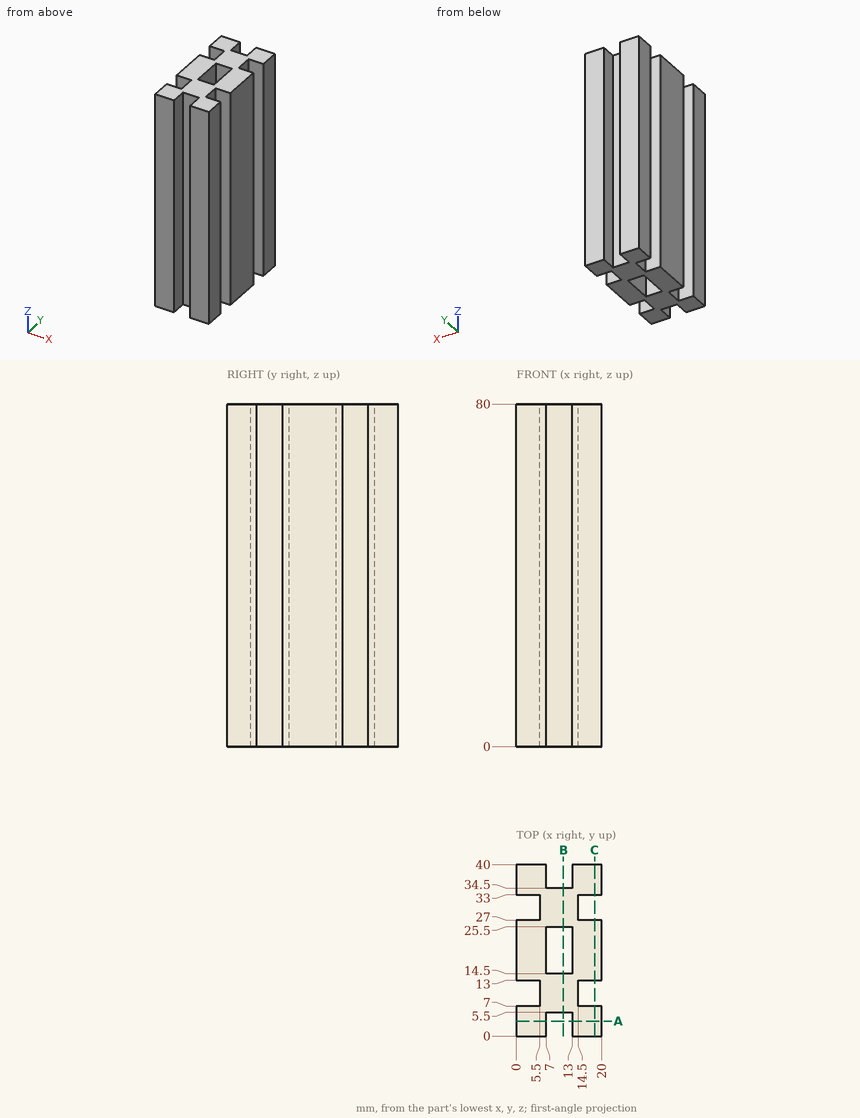
Design review of the part shown in the three views and the two pictorial views. Dimensions are in mm from the part's minimum x, y and z. Give positions to 0.01 mm unless a question says otherwise; leave off trailing zeros. Loops run counter-clockwise (first coordinate to the right, second up) from the corner with the lowest first, then second, coordinate; pieces in that order, holes last. Notation, with made-up numbers: (58.25, 86.25) -> (84.25, 86.25) arc R17 cw to (84.25, 92.25) -> close; hole circle Ø10 at (51.25, 38.5). An arc over 180 degrees is marked (long way). Write each question's results on one line, items separated by ' | '.
1) Take a section at A-A, the plane y = 3.5. Give the boundary of the cut face in (x, z), plus the area to 3 significant figures.
Conclusion:
outline: (0, 0) -> (7, 0) -> (7, 80) -> (0, 80) -> close; (13, 0) -> (20, 0) -> (20, 80) -> (13, 80) -> close | area: 1,120 mm^2
2) Insertion check: pin 1 Ø3 at (y, z) = (9.5, 39.5) entering from +X; pin 2 Ø3 at (y, z) = (11, 28) entering from -X. Each pin has a flat end and moves straight along its axis. Give the tip position at first contact, or say it passes through.
Conclusion:
pin 1: stops at x = 14.5 | pin 2: stops at x = 5.5
3) Take a section at B-B, the plane x = 11. Give the boundary of the cut face in (y, z), plus the area to 3 significant figures.
Conclusion:
outline: (5.5, 0) -> (14.5, 0) -> (14.5, 80) -> (5.5, 80) -> close; (25.5, 0) -> (34.5, 0) -> (34.5, 80) -> (25.5, 80) -> close | area: 1,440 mm^2
4) For line 1 along Y through (x, z) = (17.5, 71); line 2 along X through (y, z) = (19, 69); line 3 along Y through (x, z) = (8.5, 61), list the stretches that pass through material, from the lowest coordinate up. Write a range as from..to.
Conclusion:
line 1: y = 0..7, 13..27, 33..40 | line 2: x = 0..7, 13..20 | line 3: y = 5.5..14.5, 25.5..34.5
5) Take a section at C-C, the plane x = 18.25. Give the boundary of the cut face in (y, z), plus the area to 3 significant figures.
Conclusion:
outline: (0, 0) -> (7, 0) -> (7, 80) -> (0, 80) -> close; (13, 0) -> (27, 0) -> (27, 80) -> (13, 80) -> close; (33, 0) -> (40, 0) -> (40, 80) -> (33, 80) -> close | area: 2,240 mm^2
